```python
from build123d import *

# Parameters (mm, degrees)
SKETCH1_W                          = 50.8
SKETCH1_H                          = 50.8
BOSS_EXTRUDE1_DEPTH                = 6.35
F_1_2_0_5_DIAMETER_HOLE1_D         = 12.7
F_1_2_0_5_DIAMETER_HOLE1_DEPTH     = 70.104
F_1_2_0_5_DIAMETER_HOLE1_TIP       = 3.815464931
F_3_16_0_1875_DIAMETER_HOLE1_D     = 4.7625
F_3_16_0_1875_DIAMETER_HOLE1_DEPTH = 70.104
F_3_16_0_1875_DIAMETER_HOLE1_TIP   = 1.430799349
F_29_0_136_DIAMETER_HOLE1_D        = 3.4544
F_29_0_136_DIAMETER_HOLE1_DEPTH    = 70.104
F_29_0_136_DIAMETER_HOLE1_TIP      = 1.037806461
F_10_32_TAPPED_HOLE1_D             = 4.0386
F_10_32_TAPPED_HOLE1_DEPTH         = 11.938
F_10_32_TAPPED_HOLE1_TIP           = 1.213317848


with BuildPart() as part:
    # Sketch1 → Boss-Extrude1 (new body)
    with BuildSketch(Plane(origin=(0, 0, 0), x_dir=(0, 0, -1), z_dir=(1, 0, 0))):
        Rectangle(SKETCH1_W, SKETCH1_H)
    extrude(amount=BOSS_EXTRUDE1_DEPTH)

    # 1/2 (0.5) Diameter Hole1
    with Locations(Plane(origin=(6.35, 0, 0), x_dir=(0, 0, -1), z_dir=(1, 0, 0))):
        with Locations((0, -13.97)):
            Hole(F_1_2_0_5_DIAMETER_HOLE1_D / 2, depth=F_1_2_0_5_DIAMETER_HOLE1_DEPTH)
            with Locations((0, 0, -(F_1_2_0_5_DIAMETER_HOLE1_DEPTH + F_1_2_0_5_DIAMETER_HOLE1_TIP / 2))):  # 118° drill point
                Cone(0, F_1_2_0_5_DIAMETER_HOLE1_D / 2, F_1_2_0_5_DIAMETER_HOLE1_TIP, mode=Mode.SUBTRACT)

    # 3/16 (0.1875) Diameter Hole1
    with Locations(Plane(origin=(6.35, 0, 0), x_dir=(0, 0, -1), z_dir=(1, 0, 0))):
        with Locations((0, 12.2301)):
            Hole(F_3_16_0_1875_DIAMETER_HOLE1_D / 2, depth=F_3_16_0_1875_DIAMETER_HOLE1_DEPTH)
            with Locations((0, 0, -(F_3_16_0_1875_DIAMETER_HOLE1_DEPTH + F_3_16_0_1875_DIAMETER_HOLE1_TIP / 2))):  # 118° drill point
                Cone(0, F_3_16_0_1875_DIAMETER_HOLE1_D / 2, F_3_16_0_1875_DIAMETER_HOLE1_TIP, mode=Mode.SUBTRACT)

    # #29 (0.136) Diameter Hole1
    with Locations(Plane(origin=(6.35, 0, 0), x_dir=(0, 0, -1), z_dir=(1, 0, 0))):
        with Locations((21, 12.2301), (-21, 11.74145915)):
            Hole(F_29_0_136_DIAMETER_HOLE1_D / 2, depth=F_29_0_136_DIAMETER_HOLE1_DEPTH)
            with Locations((0, 0, -(F_29_0_136_DIAMETER_HOLE1_DEPTH + F_29_0_136_DIAMETER_HOLE1_TIP / 2))):  # 118° drill point
                Cone(0, F_29_0_136_DIAMETER_HOLE1_D / 2, F_29_0_136_DIAMETER_HOLE1_TIP, mode=Mode.SUBTRACT)

    # #10-32 Tapped Hole1
    with Locations(Plane(origin=(-0.669296778, 7.980106856, -25.4), x_dir=(-1, 0, 0), z_dir=(0, 0, -1))):
        with Locations((-3.844296778, -27.030106856), (-3.844296778, 11.069893144)):
            Hole(F_10_32_TAPPED_HOLE1_D / 2, depth=F_10_32_TAPPED_HOLE1_DEPTH)
            with Locations((0, 0, -(F_10_32_TAPPED_HOLE1_DEPTH + F_10_32_TAPPED_HOLE1_TIP / 2))):  # 118° drill point
                Cone(0, F_10_32_TAPPED_HOLE1_D / 2, F_10_32_TAPPED_HOLE1_TIP, mode=Mode.SUBTRACT)


solid = part.part
```
The listing builds one solid part. Answer for the finished solid, in the listing's coordinates (mm). A direction names the side the tool comes from. Round coordinates to 2 decimals unless told otherwise and drop trailing zeros. Write each loop counter-clockwise with the first axis right and the second up, starting at its lowest first coordinate (ties: lowest second). Pieces come first, ordered by that corner, then holes. Notation, with made-up numbers: (83.25, -9.75) -> (102.25, -9.75) arc R26 ccw to (102.25, 17.25) -> close; hole circle Ø3 at (62.5, 75.25). An arc over 180 degrees is marked (long way). Write item = value, one per line.
1) Given pin 1 (3 mm diameter, centred on x = 3.175, y = 19.05, fed in from -Z), flat-ended and moving along its own axis, determine where the tip first touches the part or whether it passes through.
Check values:
pin_1 = -13.15
2) For a pull along Y with two mould halves and no side action, classify faces 3 (the flat face through (6.35, 0, 0)), 4 (the flat face through (3, -25.4, 0)), 5 (the cylindrical face through (2.91, -17.05, -19.35)) as released by +Y, released by -Y, zero draft, split by the parting line, or undercut.
Check values:
face_3 = zero draft
face_4 = released by -Y
face_5 = undercut
3) Section C-C on y = -13.97 is taken. Write down the section's boundary in (x, z).
Check values:
outline = (0, -25.4) -> (6.35, -25.4) -> (6.35, -6.35) -> (0, -6.35) -> close; (0, 6.35) -> (6.35, 6.35) -> (6.35, 25.4) -> (0, 25.4) -> close
4) Which of the six approach directions +Z, -Z, +X, -X, +Y, -Y give full straight-line access (tool end or side, diameter ignored) to faces 1 (the flat face through (3, 0, 25.4)), 2 (the cylindrical face through (2.74, 17.08, -19.35))?
Check values:
face_1 = +Z, +X, -X, +Y, -Y
face_2 = -Z
5) Section D-D on z = 21 is taken. Write down the section's boundary in (x, y).
Check values:
outline = (0, -25.4) -> (6.35, -25.4) -> (6.35, 10.01) -> (0, 10.01) -> close; (0, 13.47) -> (6.35, 13.47) -> (6.35, 25.4) -> (0, 25.4) -> close
6) Section A-A on z = -21 is taken. Write down the section's boundary in (x, y) (3 decimals).
Check values:
outline = (0, -25.4) -> (6.35, -25.4) -> (6.35, 10.503) -> (0, 10.503) -> close; (0, 13.957) -> (6.35, 13.957) -> (6.35, 25.4) -> (0, 25.4) -> close; hole circle Ø4.039 at (3.175, -19.05); hole circle Ø4.039 at (3.175, 19.05)
7) Section B-B on z = 0 is taken. Write down the section's boundary in (x, y), plus the area to 3 significant figures.
Check values:
outline = (0, -25.4) -> (6.35, -25.4) -> (6.35, -20.32) -> (0, -20.32) -> close; (0, -7.62) -> (6.35, -7.62) -> (6.35, 9.85) -> (0, 9.85) -> close; (0, 14.61) -> (6.35, 14.61) -> (6.35, 25.4) -> (0, 25.4) -> close
area = 212 mm²
8) Straight lines are drawn through the part: line 1 along Y through (x, z) = (4, 0); line 2 along X through (y, z) = (-19.05, -20); line 3 along Z through (x, y) = (3, 12.5). For each, find the intervals that lie inside material, in ascending order. Write a range as [from, to].
Check values:
line_1 = [-25.4, -20.32], [-7.62, 9.85], [14.61, 25.4]
line_2 = [0, 1.16], [5.19, 6.35]
line_3 = [-25.4, -22.71], [-19.29, -2.37], [2.37, 19.45], [22.55, 25.4]
